The listing builds one solid part. Answer for the finished solid, in the listing's coordinates (mm). A direction names the side the tool comes from. Coordinates: 2 decimals unless noted, no trailing zeros. Loops run counter-clockwise (first coordinate to the right, second up) from the corner with the lowest first, then second, coordinate; pieces in that order, holes last. Notation, with made-up numbers: M 75.5,70 L 134.5,70 A9 ccw 134.5,75 Z; hole C 4,33 d5. An arc over 180 degrees is marked long. Return JSON: item names as keys, results as strings. Group by question number.
1. Section A-A (y = 137) is taken. Write down the section's boundary in (x, z).
2. Straight lines are drawn through the part: L1, parallel to Y at x = -38, z = -61; L2, parallel to X at y = 162.5, z = 0; L3, parallel to Z at x = -9, y = 26.5. For each, find the intervals that lie inside material, in ascending order. Write a range as from..to.
3. The mould has two halves that part along X. Classify faces 5 (the face through (-59.94, 4.93, -2.64)), 6 (the face through (-70.42, 84, 0)), 7 (the face through (-67.42, 84, 0)), 8 (the face through (-60.47, 164.93, 46.367)): pulls with the +X half, pulls with the -X half, needs draft (parallel to the pull), parting line crosses it, or undercut.
4. Which of the six approach directions +Z, -Z, +X, -X, +Y, -Y give full straight-line access (tool end or side, diameter ignored) to faces 1 (the face through (0, 84, 67.42)), 2 (the face through (0, 84, -70.42)), 3 (the face through (0, 84, 70.42)), 4 (the face through (-70.42, 229, 0))?
5. Section B-B (x = 53) is taken. Write down the section's boundary in (y, z), then the cut area to 3 significant figures.
6. Given P1, Ø0.9, axis at x = -69.5, y = 78.5, coming from the -Z side; P2, Ø1.5, axis at y = 254.5, z = 68.5, coming from the -X side; P3, Ø24, axis at y = 104.5, z = -1, coming from the -X side, each flat-ended and moving along its own axis, determine where each tip first touches the part or whether it passes through.
7. Section C-C (z = -56.5) is taken. Write down the section's boundary in (x, y).
```python
from build123d import *

# Parameters (mm, degrees)
ESQUISSE1_R                  = 76.2
ESQUISSE1_R_2                = 60
BOSS_EXTRU_1_DEPTH           = 10
ESQUISSE2_W                  = 30
ESQUISSE2_H                  = 3
BOSS_EXTRU_2_DEPTH           = 290
R_P_TITION_CIRCULAIRE1_COUNT = 4
ESQUISSE5_R                  = 76.2
ESQUISSE5_R_2                = 62.5
BOSS_EXTRU_3_DEPTH           = 10
R_P_TITION_LIN_AIRE2_COUNT   = 2
R_P_TITION_LIN_AIRE2_PITCH   = 130


with BuildPart() as part:
    # Esquisse1 → Boss.-Extru.1 (new body)
    with BuildSketch(Plane(origin=(0, 0, 0), x_dir=(1, 0, 0), z_dir=(0, 1, 0))):
        Circle(ESQUISSE1_R)
        Circle(ESQUISSE1_R_2, mode=Mode.SUBTRACT)
    extrude(amount=BOSS_EXTRU_1_DEPTH)

    # Esquisse2 → Boss.-Extru.2 (add)
    with BuildSketch(Plane(origin=(0, 10, 0), x_dir=(1, 0, 0), z_dir=(0, 1, 0))):
        with Locations((0, 68.920167566)):
            Rectangle(ESQUISSE2_W, ESQUISSE2_H)
    boss_extru_2 = extrude(amount=BOSS_EXTRU_2_DEPTH)

    # Répétition circulaire1: Boss.-Extru.2 ×4 about axis
    r_p_tition_circulaire1_axis = Axis((0, 0, 0), (0, 1, 0))
    for i in range(1, R_P_TITION_CIRCULAIRE1_COUNT):
        add(boss_extru_2.rotate(r_p_tition_circulaire1_axis, i * 360 / R_P_TITION_CIRCULAIRE1_COUNT))

    # Esquisse5 → Boss.-Extru.3 (add)
    with BuildSketch(Plane(origin=(0, 160, 0), x_dir=(1, 0, 0), z_dir=(0, 1, 0))):
        Circle(ESQUISSE5_R)
        Circle(ESQUISSE5_R_2, mode=Mode.SUBTRACT)
    boss_extru_3 = extrude(amount=BOSS_EXTRU_3_DEPTH)

    # Répétition linéaire2: Boss.-Extru.3 ×2
    with Locations(*[(0, i * R_P_TITION_LIN_AIRE2_PITCH, 0) for i in range(1, R_P_TITION_LIN_AIRE2_COUNT)]):
        add(boss_extru_3)


solid = part.part
```
Worked out:
{
 "1": {"outline": "M -70.42,-15 L -67.42,-15 L -67.42,15 L -70.42,15 Z; M -15,-70.42 L 15,-70.42 L 15,-67.42 L -15,-67.42 Z; M -15,67.42 L 15,67.42 L 15,70.42 L -15,70.42 Z; M 67.42,-15 L 70.42,-15 L 70.42,15 L 67.42,15 Z"},
 "2": {"L1": "0..10, 160..170, 290..300", "L2": "-76.2..-62.5, 62.5..76.2", "L3": "-70.42..-67.42, 67.42..70.42"},
 "3": {"face 5": "undercut", "face 6": "pulls with the -X half", "face 7": "undercut", "face 8": "parting line crosses it"},
 "4": {"face 1": "+X, -X", "face 2": "-Z, +X, -X", "face 3": "+Z, +X, -X", "face 4": "+Z, -Z, -X"},
 "5": {"outline": "M 0,-54.75 L 10,-54.75 L 10,-28.12 L 0,-28.12 Z; M 0,28.12 L 10,28.12 L 10,54.75 L 0,54.75 Z; M 160,-54.75 L 170,-54.75 L 170,-33.12 L 160,-33.12 Z; M 160,33.12 L 170,33.12 L 170,54.75 L 160,54.75 Z; M 290,-54.75 L 300,-54.75 L 300,-33.12 L 290,-33.12 Z; M 290,33.12 L 300,33.12 L 300,54.75 L 290,54.75 Z", "area": "1,400 mm^2"},
 "6": {"P1": "z = -15", "P2": "x = -15", "P3": "x = -70.42"},
 "7": {"outline": "M -51.13,0 L -20.19,0 L -20.19,10 L -51.13,10 Z; M -51.13,160 L -26.72,160 L -26.72,170 L -51.13,170 Z; M -51.13,290 L -26.72,290 L -26.72,300 L -51.13,300 Z; M 20.19,0 L 51.13,0 L 51.13,10 L 20.19,10 Z; M 26.72,160 L 51.13,160 L 51.13,170 L 26.72,170 Z; M 26.72,290 L 51.13,290 L 51.13,300 L 26.72,300 Z"}
}
